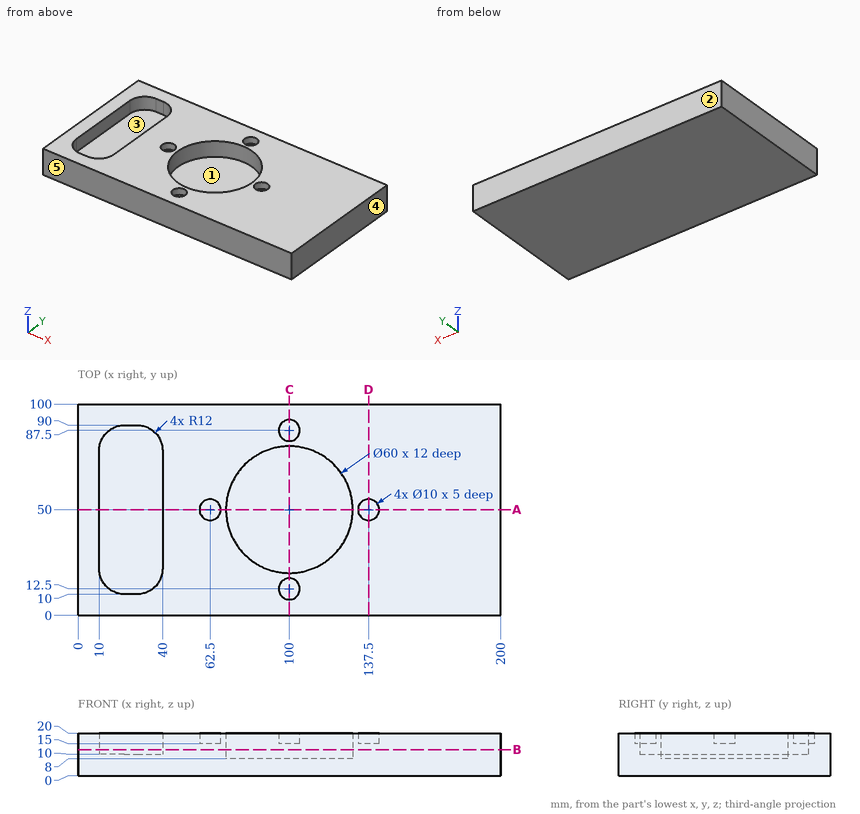
Verification items for this drawing (mm, ordinates from the low corner). A direction names the side the tool comes from. Round coordinates to 2 decimals unless told otherwise and drop trailing zeros. Order: outer loops, then holes, each group sorted by start corner. A loop starts at its lowest first (then second) coordinate and runs counter-clockwise, first axis right, second up. Notation, with made-up numbers: (7, 67.25) - (65, 67.25) arc R11 ccw to (65, 84.25) - close; hole circle Ø4 at (-27, 22.25). An arc over 180 degrees is marked (long way). Use CSV: the item, a comma, the result in double quotes.
(1) Mould release check, pull along X, two halves, no side actions. Record for the marked faces 3, 4 and 5: released by +X, released by -X, zero draft, split by the parting line, or undercut.
Entries:
face 3,"undercut"
face 4,"released by +X"
face 5,"zero draft"
(2) Section check A-A on y = 50. Record the boundary of the cut face in (x, z).
Entries:
outline,"(0, 0) - (200, 0) - (200, 20) - (142.5, 20) - (142.5, 15) - (132.5, 15) - (132.5, 20) - (130, 20) - (130, 8) - (70, 8) - (70, 20) - (67.5, 20) - (67.5, 15) - (57.5, 15) - (57.5, 20) - (40, 20) - (40, 10) - (10, 10) - (10, 20) - (0, 20) - close"
(3) Section check C-C on x = 100. Record the boundary of the cut face in (y, z).
Entries:
outline,"(0, 0) - (100, 0) - (100, 20) - (92.5, 20) - (92.5, 15) - (82.5, 15) - (82.5, 20) - (80, 20) - (80, 8) - (20, 8) - (20, 20) - (17.5, 20) - (17.5, 15) - (7.5, 15) - (7.5, 20) - (0, 20) - close"
(4) Section check D-D on x = 137.5. Record the boundary of the cut face in (y, z).
Entries:
outline,"(0, 0) - (100, 0) - (100, 20) - (55, 20) - (55, 15) - (45, 15) - (45, 20) - (0, 20) - close"
(5) Gauge pin test, flat ends, axial feed: pin 1 Ø8 at (x, y) = (62.5, 50.5) entering from +Z; pin 2 Ø15 at (x, y) = (27.5, 52) entering from +Z. Record the tip position at first contact, or that the pin passes through.
Entries:
pin 1,"z = 15"
pin 2,"z = 10"
(6) Thickness scan on probe 1 along Y at (x, z) = (137.5, 16.3); probe 2 along X at (y, z) = (52.5, 17); probe 3 along X at (y, z) = (17, 16). Record the ranges inside material, lowest first. Write a range as from..to.
Entries:
probe 1,"0..45, 55..100"
probe 2,"0..10, 40..58.17, 66.83..70.1, 129.9..133.17, 141.83..200"
probe 3,"0..11.09, 38.91..97.82, 102.18..200"
(7) Section check B-B on z = 12.25. Record the boundary of the cut face in (x, y), and give its area (3 significant figures).
Entries:
outline,"(0, 0) - (200, 0) - (200, 100) - (0, 100) - close; hole (10, 22) arc R12 ccw to (22, 10) - (28, 10) arc R12 ccw to (40, 22) - (40, 78) arc R12 ccw to (28, 90) - (22, 90) arc R12 ccw to (10, 78) - close; hole circle Ø60 at (100, 50)"
area,"14,900 mm^2"
(8) Access from +Z, -Z, +X, -X, +Y, -Y to the whole of each face (thin tool, end or side, straight path). Record for the marked faces 1 and 2.
Entries:
face 1,"+Z"
face 2,"+Z, -Z, +X, -X, +Y"
